```python
from build123d import *

# Parameters (mm, degrees)
ENLEV_MAT_EXTRU1_DEPTH = 1.3
ESQUISSE3_W            = 1.5
ESQUISSE3_H            = 10
CHANFREIN1_SIZE        = 0.3


with BuildPart() as part:
    # Esquisse1 → Base-R_volution (revolve)
    with BuildSketch(Plane(origin=(0, 0, 0), x_dir=(1, 0, 0), z_dir=(0, 1, 0)), mode=Mode.PRIVATE) as base_r_volution_sk:
        with BuildLine():
            Line((0, 0), (2.75, 0))
            Line((2.75, 0), (2.75, 2.7))
            ThreePointArc((2.75, 2.7), (2.662132034, 2.912132034), (2.45, 3))
            Line((2.45, 3), (0, 3))
            Line((0, 3), (0, 0))
        make_face()
    revolve(base_r_volution_sk.sketch.rotate(Axis((0, 0, 0), (0, 0, -1)), 180), axis=Axis((0, 0, 0), (0, 0, -1)))

    # Esquisse2 → enlev-mat-Extru1 (cut)
    with BuildSketch(Plane.XY.offset(-3)):
        Polygon((1.25, -0.721687836), (1.25, 0.721687836), (0, 1.443375673), (-1.25, 0.721687836), (-1.25, -0.721687836), (0, -1.443375673), align=None)
    extrude(amount=ENLEV_MAT_EXTRU1_DEPTH, mode=Mode.SUBTRACT)

    # Esquisse3 → Boss.-R_vol.1 (revolve)
    with BuildSketch(Plane(origin=(0, 0, 0), x_dir=(1, 0, 0), z_dir=(0, 1, 0))):
        with Locations((0.75, -5)):
            Rectangle(ESQUISSE3_W, ESQUISSE3_H)
    revolve(axis=Axis((0, 0, 0), (0, 0, 1)))

    # Chanfrein1
    chanfrein1_edges = [part.edges().sort_by_distance(p)[0] for p in [
        (-1.5, 0, 10),
    ]]
    chamfer(chanfrein1_edges, length=CHANFREIN1_SIZE)


solid = part.part
```
Could you check a few things on this model? Use its own coordinates, in mm. A direction names the side the tool comes from. Round coordinates to 2 decimals unless told otherwise and drop trailing zeros. Loops run counter-clockwise (first coordinate to the right, second up) from the corner with the lowest first, then second, coordinate; pieces in that order, holes last.
Q1. For P1, Ø1.5, axis at x = 2, z = 1.5, coming from the +Y side; P2, Ø1.5, axis at x = 2, z = 8.5, coming from the -Y side; P3, Ø1.2, axis at x = 0.5, y = 0, coming from the -Z side, each with a flat end and sliding along its axis, tell me the tip position at first contact or that it passes through.
Q2. Thinking about a two-plate mould opening in X: for faces 4 (the cylindrical face through (-1.5, 0.07, 4.78)), 5 (the flat face through (-1.1, -1.1, -3)), 6 (the flat face through (1.25, 0, -2)), which applies, pulls with the +X half, pulls with the -X half, needs draft (parallel to the pull), parting line crosses it, or undercut?
Q3. On a 3-axis mill with a long thin cutter (end or side, diameter ignored), from which of +Z, -Z, +X, -X, +Y, -Y can I reach the whole of each face in a straight line? I mean faces 1 (the cylindrical face through (0.596, -2.685, -1.369)), 2 (the flat face through (1.2, -1.2, 0)), 3 (the flat face through (0.63, 1.08, -2.36)). Say none if no direction works.
Q4. I want a section at C-C (z = -1). Write out the boundary of the cut face in (x, y), and give its area (3 significant figures).
Q5. Please list where these lines run through material, in increasing order: L1, parallel to X at y = -0.05, z = 0.5; L2, parallel to Z at x = -0.55, y = 1.75; L3, parallel to Y at x = 2, z = -1.5.
Q6. I want a section at B-B (z = 8). Write out the boundary of the cut face in (x, y), and give its area (3 significant figures).
Q7. I want a section at A-A (y = 0). Write out the boundary of the cut face in (x, z).
Answer below:
1. P1: stops at y = 0.83
1. P2: stops at y = -0.83
1. P3: stops at z = -1.7
2. face 4: parting line crosses it
2. face 5: needs draft
2. face 6: undercut
3. face 1: +Z, -Z
3. face 2: +Z
3. face 3: -Z
4. outline: circle Ø5.5 at (0, 0)
4. area: 23.8 mm2
5. L1: x = -1.5 to 1.5
5. L2: z = -3 to 0
5. L3: y = -1.89 to 1.89
6. outline: circle Ø3 at (0, 0)
6. area: 7.07 mm2
7. outline: (-2.75, -2.7) arc R0.3 ccw to (-2.45, -3) - (-1.25, -3) - (-1.25, -1.7) - (1.25, -1.7) - (1.25, -3) - (2.45, -3) arc R0.3 ccw to (2.75, -2.7) - (2.75, 0) - (1.5, 0) - (1.5, 9.7) - (1.2, 10) - (-1.2, 10) - (-1.5, 9.7) - (-1.5, 0) - (-2.75, 0) - close
